```python
from build123d import *

# Parameters (mm, degrees)
CROQUIS1_W              = 90
CROQUIS1_H              = 90
SALIENTE_EXTRUIR2_DEPTH = 15
CROQUIS2_R              = 10
SALIENTE_EXTRUIR3_DEPTH = 60
SALIENTE_EXTRUIR4_DEPTH = 1
REDONDEO1_R             = 5
REDONDEO2_R             = 5
REDONDEO3_R             = 5
REDONDEO4_R             = 10


with BuildPart() as part:
    # Croquis1 → Saliente-Extruir2 (new body)
    with BuildSketch(Plane.XY):
        Rectangle(CROQUIS1_W, CROQUIS1_H)
    extrude(amount=SALIENTE_EXTRUIR2_DEPTH)

    # Croquis2 → Saliente-Extruir3 (add)
    with BuildSketch(Plane(origin=(0, 0, 0), x_dir=(-1, 0, 0), z_dir=(0, 0, -1))):
        Circle(CROQUIS2_R)
    extrude(amount=SALIENTE_EXTRUIR3_DEPTH)

    # Croquis3 → Saliente-Extruir4 (add)
    with BuildSketch(Plane.XY.offset(15)):
        Polygon((10.5, 0.5), (10.5, 2.5), (11.5, 2.5), (11.5, 0.5), (21.5, 0.5), (21.5, 2.5), (22.5, 2.5), (22.5, 0.5), (32.5, 0.5), (32.5, 2.5), (33.5, 2.5), (33.5, 0.5), (43.5, 0.5), (41.378679656, 2.621320344), (42.378679656, 2.621320344), (44.5, 0.5), (44.5, -0.5), (42.378679656, -2.621320344), (41.378679656, -2.621320344), (43.5, -0.5), (33.5, -0.5), (33.5, -2.5), (32.5, -2.5), (32.5, -0.5), (22.5, -0.5), (22.5, -2.5), (21.5, -2.5), (21.5, -0.5), (11.5, -0.5), (11.5, -2.5), (10.5, -2.5), (10.5, -0.5), (0.5, -0.5), (0.5, -10.5), (2.5, -10.5), (2.5, -11.5), (0.5, -11.5), (0.5, -21.5), (2.5, -21.5), (2.5, -22.5), (0.5, -22.5), (0.5, -32.5), (2.5, -32.5), (2.5, -33.5), (0.5, -33.5), (0.5, -43.5), (2.621320344, -41.378679656), (2.621320344, -42.378679656), (0.5, -44.5), (-0.5, -44.5), (-2.621320344, -42.378679656), (-2.621320344, -41.378679656), (-0.5, -43.5), (-0.5, -33.5), (-2.5, -33.5), (-2.5, -32.5), (-0.5, -32.5), (-0.5, -22.5), (-2.5, -22.5), (-2.5, -21.5), (-0.5, -21.5), (-0.5, -11.5), (-2.5, -11.5), (-2.5, -10.5), (-0.5, -10.5), (-0.5, -0.5), (-10.5, -0.5), (-10.5, -2.5), (-11.5, -2.5), (-11.5, -0.5), (-21.5, -0.5), (-21.5, -2.5), (-22.5, -2.5), (-22.5, -0.5), (-32.5, -0.5), (-32.5, -2.5), (-33.5, -2.5), (-33.5, -0.5), (-43.5, -0.5), (-41.378679656, -2.621320344), (-42.378679656, -2.621320344), (-44.5, -0.5), (-44.5, 0.5), (-42.378679656, 2.621320344), (-41.378679656, 2.621320344), (-43.5, 0.5), (-33.5, 0.5), (-33.5, 2.5), (-32.5, 2.5), (-32.5, 0.5), (-22.5, 0.5), (-22.5, 2.5), (-21.5, 2.5), (-21.5, 0.5), (-11.5, 0.5), (-11.5, 2.5), (-10.5, 2.5), (-10.5, 0.5), (-0.5, 0.5), (-0.5, 10.5), (-2.5, 10.5), (-2.5, 11.5), (-0.5, 11.5), (-0.5, 21.5), (-2.5, 21.5), (-2.5, 22.5), (-0.5, 22.5), (-0.5, 32.5), (-2.5, 32.5), (-2.5, 33.5), (-0.5, 33.5), (-0.5, 43.5), (-2.621320344, 41.378679656), (-2.621320344, 42.378679656), (-0.5, 44.5), (0.5, 44.5), (2.621320344, 42.378679656), (2.621320344, 41.378679656), (0.5, 43.5), (0.5, 33.5), (2.5, 33.5), (2.5, 32.5), (0.5, 32.5), (0.5, 22.5), (2.5, 22.5), (2.5, 21.5), (0.5, 21.5), (0.5, 11.5), (2.5, 11.5), (2.5, 10.5), (0.5, 10.5), (0.5, 0.5), align=None)
    extrude(amount=SALIENTE_EXTRUIR4_DEPTH)

    # Redondeo1
    redondeo1_edges = [part.edges().sort_by_distance(p)[0] for p in [
        (45, -45, 7.5),
        (-45, -45, 7.5),
        (-45, 45, 7.5),
        (45, 45, 7.5),
    ]]
    fillet(redondeo1_edges, radius=REDONDEO1_R)

    # Redondeo2
    redondeo2_edges = [part.edges().sort_by_distance(p)[0] for p in [
        (0, -45, 0),
        (45, 0, 0),
        (-45, 0, 0),
        (0, 45, 0),
        (43.535533906, 43.535533906, 0),
        (-43.535533906, 43.535533906, 0),
        (43.535533906, -43.535533906, 0),
        (-43.535533906, -43.535533906, 0),
    ]]
    fillet(redondeo2_edges, radius=REDONDEO2_R)

    # Redondeo3
    redondeo3_edges = [part.edges().sort_by_distance(p)[0] for p in [
        (10, 0, 0),
    ]]
    fillet(redondeo3_edges, radius=REDONDEO3_R)

    # Redondeo4
    redondeo4_edges = [part.edges().sort_by_distance(p)[0] for p in [
        (10, 0, -60),
    ]]
    fillet(redondeo4_edges, radius=REDONDEO4_R)


solid = part.part
```
The listing builds one solid part. Answer for the finished solid, in the listing's coordinates (mm). A direction names the side the tool comes from. Coordinates: 2 decimals unless noted, no trailing zeros. Loops run counter-clockwise (first coordinate to the right, second up) from the corner with the lowest first, then second, coordinate; pieces in that order, holes last. Notation, with made-up numbers: (-13, 40) -> (1, 40) arc R23 cw to (1, 73) -> close; hole circle Ø3 at (83.5, 22). An arc over 180 degrees is marked (long way). Return JSON: item names as keys, results as strings. Group by question number.
(1) A cutting plane is placed at B-B on z = -32.5. Write down the section's boundary in (x, y), and give its area (3 significant figures).
(2) Which of the six approach directions +Z, -Z, +X, -X, +Y, -Y give full straight-line access (tool end or side, diameter ignored) to faces 1 (the flat face through (45, -1, 10)), 2 (the flat face through (17, 1, 0))?
(3) Find the intervals of material crossed by probe 1 along Z at (x, y) = (39, 25); probe 2 along Z at (x, y) = (-4, 12); probe 3 along X at (y, z) = (4, -34), in increasing order. Write a range as from..to.
(4) A cutting plane is placed at A-A on x = 24. Write down the section's boundary in (y, z), and give its area (3 significant figures).
(5) Determine the mould class of faces 3 (the cylindrical face through (2.17, -9.76, -27.18)), 4 (the flat face through (-45, -1, 10)), 5 (the cylindrical face through (43, 44, 10)), 6 (the cylindrical face through (1, -43, 1)) for opening direction Y: released by +Y, released by -Y, zero draft, split by the parting line, or undercut.
(6) Given pin 1 Ø0.8 at (x, z) = (-1, 15.5) entering from -Y; pin 2 Ø12 at (y, z) = (-2.5, -14.5) entering from +X; pin 3 Ø0.5 at (y, z) = (40, 15.5) entering from +X, each flat-ended and moving along its own axis, determine where each tip first touches the part or whether it passes through.
The answers:
{
 "1": {"outline": "circle Ø20 at (0, 0)", "area": "314 mm^2"},
 "2": {"face 1": "+Z, -Z, +X, +Y, -Y", "face 2": "-Z"},
 "3": {"probe 1": "z = 0..15", "probe 2": "z = -0.59..15", "probe 3": "x = -9.17..9.17"},
 "4": {"outline": "(-45, 5) arc R5 ccw to (-40, 0) -> (40, 0) arc R5 ccw to (45, 5) -> (45, 15) -> (0.5, 15) -> (0.5, 16) -> (-0.5, 16) -> (-0.5, 15) -> (-45, 15) -> close", "area": "1,340 mm^2"},
 "5": {"face 3": "split by the parting line", "face 4": "zero draft", "face 5": "released by +Y", "face 6": "released by -Y"},
 "6": {"pin 1": "stops at y = -44.4", "pin 2": "stops at x = 10", "pin 3": "stops at x = 0.5"}
}
